```python
from build123d import *

# Parameters (mm, degrees)
F0_W     = 20
F0_H     = 15.25
F0_H_2   = 7.5
F1_DEPTH = 10
F2_DEPTH = 3
F4_D     = 4.4
F4_DEPTH = 20
F4_TIP   = 1.3218933619


with BuildPart() as f1:
    # F0 (on Top) → F1 (new body)
    with BuildSketch(Plane.XY):
        with Locations((10, 11.375)):
            Rectangle(F0_W, F0_H)
        with Locations((-10, 11.375)):
            Rectangle(F0_W, F0_H)
        with Locations((10, -11.375)):
            Rectangle(F0_W, F0_H)
        with Locations((-10, -11.375)):
            Rectangle(F0_W, F0_H)
        with Locations((10, 0)):
            Rectangle(F0_W, F0_H_2)
        with Locations((-10, 0)):
            Rectangle(F0_W, F0_H_2)
    extrude(amount=-F1_DEPTH)

    # F0 (on Top) → F2 (join)
    with BuildSketch(Plane.XY):
        with Locations((10, 0)):
            Rectangle(F0_W, F0_H_2)
        with Locations((-10, 0)):
            Rectangle(F0_W, F0_H_2)
    extrude(amount=F2_DEPTH)

    # F4
    with Locations(Plane(origin=(0, 0, -10), x_dir=(1, 0, 0), z_dir=(0, 0, -1))):
        with Locations((0, 0)):
            Hole(F4_D / 2, depth=F4_DEPTH)
            with Locations((0, 0, -(F4_DEPTH + F4_TIP / 2))):  # 118° drill point
                Cone(0, F4_D / 2, F4_TIP, mode=Mode.SUBTRACT)


solid = f1.part
```
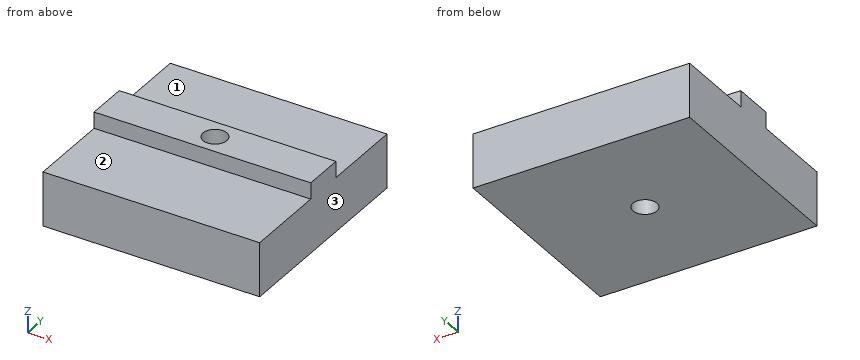
Could you check a few things on this model? Use its own coordinates, in mm. Face numbers are marked on the shaded views. A direction names the side the tool comes from. Round coordinates to 2 decimals unless told otherwise and drop trailing zeros. Loops run counter-clockwise (first coordinate to the right, second up) from the corner with the lowest first, then second, coordinate; pieces in that order, holes last. Notation, with made-up numbers: (-25.75, -26) - (16.25, -26) arc R16 cw to (16.25, -6) - close; hole circle Ø4 at (33.5, 30). An arc over 180 degrees is marked (long way). Answer as CSV lines item,"result".
1. I want a section at B-B on y = 0. List the corners of the cut face in (x, z) for me, then the cut area to 3 significant figures.
Filled in:
outline,"(-20, -10) - (-2.2, -10) - (-2.2, 3) - (-20, 3) - close; (2.2, -10) - (20, -10) - (20, 3) - (2.2, 3) - close"
area,"463 mm^2"
2. I want a section at C-C on z = 1.5. List the corners of the cut face in (x, y) for me.
Filled in:
outline,"(-20, -3.75) - (20, -3.75) - (20, 3.75) - (-20, 3.75) - close; hole circle Ø4.4 at (0, 0)"
3. On a 3-axis mill with a long thin cutter (end or side, diameter ignored), from which of +Z, -Z, +X, -X, +Y, -Y can I reach the whole of each face in a straight line? I mean the marked faces 1, 2 and 3. Say none if no direction works.
Filled in:
face 1,"+Z, +X, -X, +Y"
face 2,"+Z, +X, -X, -Y"
face 3,"+Z, -Z, +X, +Y, -Y"
4. I want a section at D-D on x = 11. List the corners of the cut face in (y, z) for me, then the cut area to 4 significant figures.
Filled in:
outline,"(-19, -10) - (19, -10) - (19, 0) - (3.75, 0) - (3.75, 3) - (-3.75, 3) - (-3.75, 0) - (-19, 0) - close"
area,"402.5 mm^2"
5. Please list where these lines run through material, in increasing order: line 1 along Y through (x, z) = (0, -4); line 2 along Z through (x, y) = (-8.5, 10); line 3 along X through (y, z) = (-2, -5). Write a range as [from, to].
Filled in:
line 1,"y = [-19, -2.2], [2.2, 19]"
line 2,"z = [-10, 0]"
line 3,"x = [-20, -0.92], [0.92, 20]"
6. For pin 1 Ø3.5 at (x, z) = (-1.5, 1.5) entering from -Y; pin 2 Ø2.5 at (x, z) = (-4, 1.5) entering from +Y; pin 3 Ø2 at (x, y) = (-14, 13.5) entering from +Z, each with a flat end and sliding along its axis, tell me the tip position at first contact or that it passes through.
Filled in:
pin 1,"stops at y = -19"
pin 2,"stops at y = 3.75"
pin 3,"stops at z = 0"
7. I want a section at A-A on x = 0. List the corners of the cut face in (y, z) for me.
Filled in:
outline,"(-19, -10) - (-2.2, -10) - (-2.2, 3) - (-3.75, 3) - (-3.75, 0) - (-19, 0) - close; (2.2, -10) - (19, -10) - (19, 0) - (3.75, 0) - (3.75, 3) - (2.2, 3) - close"
